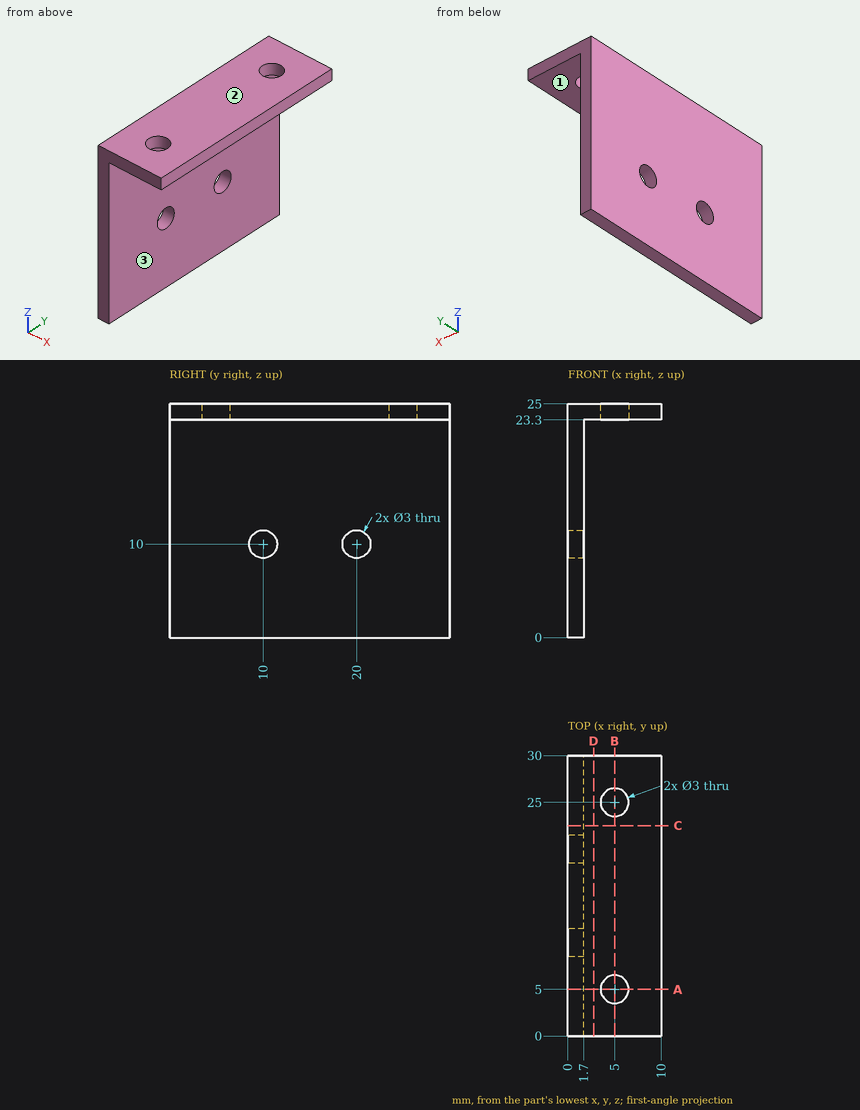
Answer from the drawing. Dimensions are ordinates in mm from the lowest x, y and z of the part. Coordinates: 2 decimals unless noted, no trailing zeros. Write each loop counter-clockwise with the first axis right and the second up, starting at its lowest first coordinate (ties: lowest second). Pieces come first, ordered by that corner, then holes. Notation, with made-up numbers: M 49.5,58.5 L 53.5,58.5 A25 cw 53.5,73.5 Z; hole C 52.25,68.25 d8. An arc over 180 degrees is marked long. Use one line per item in the form item = value. Start each with the question number.
1. The part is cut by section C-C (y = 22.5). Give the vertices of the cut face in (x, z).
2. Each of these flat-tipped pins is pushed along its axis until it touches: P1, Ø4, axis at x = 5.5, y = 14.5, coming from the -Z side; P2, Ø4, axis at y = 20, z = 10, coming from the +X side. Where does it stop, or does it pass through?
3. The part is cut by section D-D (x = 2.75). Give the vertices of the cut face in (y, z), plus the area to 3 significant figures.
4. The part is cut by section A-A (y = 5). Give the vertices of the cut face in (x, z), plus the area to 3 significant figures.
5. Straight lines are drawn through the part: probe 1 along Y at (x, z) = (5, 24.4); probe 2 along Y at (x, z) = (1.3, 10); probe 3 along Z at (x, y) = (8.75, 8.75). For each, find the intervals that lie inside material, in ascending order. Write a range as from..to.
6. The mould has two halves that part along Z. Classify the marked faces 1, 2 and 3: released by +Z, released by -Z, zero draft, split by the parting line, or undercut.
7. The part is cut by section B-B (x = 5). Give the vertices of the cut face in (y, z).
Evaluation:
q1.outline = M 0,0 L 1.7,0 L 1.7,23.3 L 10,23.3 L 10,25 L 0,25 Z
q2.P1 = 23.3
q2.P2 = 1.7
q3.outline = M 0,23.3 L 30,23.3 L 30,25 L 0,25 Z
q3.area = 51.0 mm^2
q4.outline = M 0,0 L 1.7,0 L 1.7,23.3 L 3.5,23.3 L 3.5,25 L 0,25 Z; M 6.5,23.3 L 10,23.3 L 10,25 L 6.5,25 Z
q4.area = 51.5 mm^2
q5.probe_1 = 0..3.5, 6.5..23.5, 26.5..30
q5.probe_2 = 0..8.5, 11.5..18.5, 21.5..30
q5.probe_3 = 23.3..25
q6.face_1 = released by -Z
q6.face_2 = released by +Z
q6.face_3 = zero draft
q7.outline = M 0,23.3 L 3.5,23.3 L 3.5,25 L 0,25 Z; M 6.5,23.3 L 23.5,23.3 L 23.5,25 L 6.5,25 Z; M 26.5,23.3 L 30,23.3 L 30,25 L 26.5,25 Z
